```python
from build123d import *

# Parameters (mm, degrees)
EXTRUDE_1_DEPTH        = 20
FILLET_1_R             = 2
FILLET_2_R             = 2
SKETCH_30_W            = 1.65
SKETCH_30_H            = 8
SKETCH_31_R            = 3.5
CUT_EXTRUDE_1_DEPTH    = 4
CUT_EXTRUDE_2_DEPTH    = 10
SKETCH_34_R            = 3.25
CUT_EXTRUDE_3_DEPTH    = 6
HOLE_WIZARD_M4_2_D     = 3.3
HOLE_WIZARD_M4_2_DEPTH = 4
SKETCH_38_W            = 5
SKETCH_38_H            = 10
CUT_EXTRUDE_4_DEPTH    = 11


with BuildPart() as part:
    # 草图1 → 凸台-拉伸1 (new body)
    with BuildSketch(Plane.XY):
        Polygon((0.020144186, -0.052366179), (0.016918395, 5.947632954), (-19.983081605, 5.947632954), (-20.000068427, 12.447632954), (0.03759791, 12.447632954), (0.03759791, 20.447632954), (-19.96240209, 20.447632954), (-11.597239053, 51.666846423), (-21.256497316, 54.255036874), (-30.315163894, 20.447632954), (-30.279663837, -0.052366179), align=None)
    extrude(amount=EXTRUDE_1_DEPTH)

    # 圆角1
    fillet_1_edges = [part.edges().sort_by_distance(p)[0] for p in [
        (-19.96240209, 20.447632954, 10),
    ]]
    fillet(fillet_1_edges, radius=FILLET_1_R)

    # 圆角2
    fillet_2_edges = [part.edges().sort_by_distance(p)[0] for p in [
        (-30.279663837, -0.052366179, 10),
    ]]
    fillet(fillet_2_edges, radius=FILLET_2_R)

    # 草图30 → M4 螺纹孔的螺纹孔钻头1 (revolve, cut)
    with BuildSketch(Plane(origin=(-5.798619526, 12.447632954, 10), x_dir=(0, 0, -1), z_dir=(1, 0, 0))):
        with Locations((0.825, 4)):
            Rectangle(SKETCH_30_W, SKETCH_30_H)
    revolve(axis=Axis((-5.798619526, 6.097632954, 10), (0, 1, 0)), mode=Mode.SUBTRACT)

    # 草图31 → 切除-拉伸1 (cut)
    with BuildSketch(Plane.XZ.offset(-12.447632954)):
        with Locations((-5.798619526, 10)):
            Circle(SKETCH_31_R)
    extrude(amount=-CUT_EXTRUDE_1_DEPTH, mode=Mode.SUBTRACT)

    # 草图33 → 切除-拉伸2 (cut)
    with BuildSketch(Plane.XY.offset(20)):
        Polygon((-21.256497316, 54.255036874), (-11.597239053, 51.666846423), (-14.185429504, 42.00758816), (-23.844687767, 44.595778611), align=None)
    extrude(amount=-CUT_EXTRUDE_2_DEPTH, mode=Mode.SUBTRACT)

    # 草图34 → 切除-拉伸3 (cut)
    with BuildSketch(Plane(origin=(0, 0, 0), x_dir=(-1, 0, 0), z_dir=(0, 0, -1))):
        with Locations((17.72096341, 48.131312517)):
            Circle(SKETCH_34_R)
    extrude(amount=-CUT_EXTRUDE_3_DEPTH, mode=Mode.SUBTRACT)

    # M4 螺纹孔的螺纹孔钻头2
    with Locations(Plane(origin=(0, 0, 6), x_dir=(-1, 0, 0), z_dir=(0, 0, -1))):
        with Locations((17.72096341, 48.131312517)):
            Hole(HOLE_WIZARD_M4_2_D / 2, depth=HOLE_WIZARD_M4_2_DEPTH)

    # 草图38 → 切除-拉伸4 (cut)
    with BuildSketch(Plane(origin=(-23.737082949, 6.360332207, 0), x_dir=(0, 0, -1), z_dir=(0.965925826, -0.258819045, 0))):
        with Locations((-2.5, 41.904754985)):
            Rectangle(SKETCH_38_W, SKETCH_38_H)
    extrude(amount=-CUT_EXTRUDE_4_DEPTH, mode=Mode.SUBTRACT)


solid = part.part
```
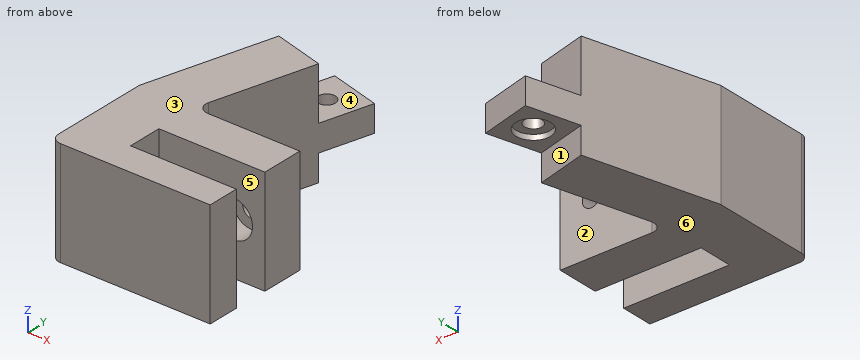
Can you work these out from the model? Positions are in its coordinate system, mm. Face numbers are marked on the shaded views. A direction names the side the tool comes from. Coordinates: 2 decimals unless noted, no trailing zeros. Write each loop counter-clockwise with the first axis right and the second up, starting at its lowest first coordinate (ties: lowest second). Pieces come first, ordered by that corner, then holes. Notation, with made-up numbers: M 42,32.5 L 80,32.5 A21 ccw 80,46.5 Z; hole C -12,88.25 d8. An arc over 180 degrees is marked long. Answer as CSV lines item,"result".
Item 1: Imagine slicing it at A-A on x = -6.5. List the corners of the cut face in (y, z) for me.
Geometry results:
outline,"M -0.05,0 L 5.95,0 L 5.95,20 L -0.05,20 Z; M 12.45,0 L 20.45,0 L 20.45,8.51 L 16.45,8.51 L 16.45,6.57 L 12.45,6.57 Z; M 12.45,13.43 L 16.45,13.43 L 16.45,11.49 L 20.45,11.49 L 20.45,20 L 12.45,20 Z"
Item 2: Imagine slicing it at D-D on x = -23. List the corners of the cut face in (y, z) for me, plus the area to 3 significant figures.
Geometry results:
outline,"M -0.05,0 L 44.37,0 L 44.37,5 L 47.75,5 L 47.75,10 L 44.37,10 L 44.37,20 L -0.05,20 Z"
area,"905 mm2"
Item 3: We'd pull the mould along Y, two halves only. Please class the marked faces 1, 2 and 3: +Y half, -Y half, draft (parallel to the pull), parting line (faces both ways), or undercut.
Geometry results:
face 1,"+Y half"
face 2,"undercut"
face 3,"draft"
Item 4: On a 3-axis mill with a long thin cutter (end or side, diameter ignored), from which of +Z, -Z, +X, -X, +Y, -Y can I reach the whole of each face in a straight line? I mean the marked faces 4, 5 and 6. Say none if no direction works.
Geometry results:
face 4,"+Z, +X, +Y"
face 5,"+Z, -Z, +X"
face 6,"-Z, +X, -X, +Y, -Y"
Item 5: Imagine slicing it at B-B on z = 16. List the corners of the cut face in (x, y) for me.
Geometry results:
outline,"M -30.32,20.45 L -30.28,1.94 A2 ccw -28.28,-0.05 L 0.02,-0.05 L 0.02,5.95 L -19.98,5.95 L -20,12.45 L 0.04,12.45 L 0.04,20.45 L -17.36,20.45 A2 cw -19.29,22.97 L -14.19,42.01 L -23.84,44.6 Z"
Item 6: I'm going to push flat-ended pins straight in: P1, Ø8.5, axis at x = -8.5, z = 6, coming from the +Y side; P2, Ø2, axis at x = -8.5, z = 12.5, coming from the +Y side; P3, Ø1, axis at y = 11.5, z = 15.5, coming from the +X side. Where does each tip first touch, or does it pass through?
Geometry results:
P1,"stops at y = 51.98"
P2,"stops at y = 20.45"
P3,"stops at x = -20"
Item 7: Imagine slicing it at C-C on x = -13.5. List the corners of the cut face in (y, z) for me.
Geometry results:
outline,"M -0.05,0 L 5.95,0 L 5.95,20 L -0.05,20 Z; M 12.45,0 L 20.45,0 L 20.45,20 L 12.45,20 Z; M 44.57,5 L 52.18,5 L 52.18,10 L 44.57,10 Z"
Item 8: Please list where these lines run through material, in increasing order: line 1 along X through (y, z) = (18.55, 10); line 2 along Y through (x, z) = (-14, 15.75); line 3 along X through (y, z) = (37, 8.75).
Geometry results:
line 1,"x = -30.31 to -7.45, -4.15 to 0.04"
line 2,"y = -0.05 to 5.95, 12.45 to 20.45"
line 3,"x = -25.88 to -15.53"
